from build123d import *

# Parameters (mm, degrees)
SKETCH1_R           = 4.7625
BOSS_EXTRUDE1_DEPTH = 12.7
SKETCH2_R           = 6.35
BOSS_EXTRUDE2_DEPTH = 50.8


with BuildPart() as part:
    # Sketch1 → Boss-Extrude1 (new body)
    with BuildSketch(Plane.XY):
        with BuildLine():
            Line((-12.7, 0), (-12.7, 127))
            Line((-12.7, 127), (12.7, 127))
            Line((12.7, 127), (12.7, 0))
            ThreePointArc((12.7, 0), (0, -12.7), (-12.7, 0))
        make_face()
        Circle(SKETCH1_R, mode=Mode.SUBTRACT)
    extrude(amount=BOSS_EXTRUDE1_DEPTH)

    # Sketch2 → Boss-Extrude2 (add)
    with BuildSketch(Plane(origin=(12.7, 0, 0), x_dir=(0, 0, -1), z_dir=(1, 0, 0))):
        with Locations((-6.35, 12.7)):
            Circle(SKETCH2_R)
    extrude(amount=BOSS_EXTRUDE2_DEPTH)


solid = part.part
Work out the finished part from the listing and answer in its coordinate system (mm). A direction names the side the tool comes from. Give positions to 0.01 mm unless a question says otherwise; leave off trailing zeros. Write each loop counter-clockwise with the first axis right and the second up, starting at its lowest first coordinate (ties: lowest second). Pieces come first, ordered by that corner, then holes. Notation, with made-up numbers: (27, 88.25) - (36, 88.25) arc R31 cw to (36, 119.25) - close; hole circle Ø11 at (14.25, 57.5). An arc over 180 degrees is marked (long way). One line per item, written item: value. Start each with the question number.
1. Consider probe 1 along Y at (x, z) = (0, 5.25); probe 2 along Y at (x, z) = (0.5, 4.75); probe 3 along X at (y, z) = (110.5, 3.5). Determine where each line is inside the solid, lowest interval first.
2. For a pull along X with two mould halves and no side action, classify faces 3 (the flat face through (12.7, 4, 6)), 4 (the flat face through (-12.7, 63, 6)), 5 (the cylindrical face through (-3.78, -2.9, 6.26)), 6 (the flat face through (0, 58, 12.7)) as +X half, -X half, draft (parallel to the pull), parting line (faces both ways), or undercut.
3. For faces 1 (the cylindrical face through (37.744, 18.054, 2.936)), 2 (the flat face through (63.5, 13, 6)), determine the directions among +Z, -Z, +X, -X, +Y, -Y from which every point of the face is accessible in a straight line to the end or side of a thin tool.
4. Find section D-D (y = 80). Write down the section's boundary in (x, z).
5. Find section C-C (y = -1.5). Write down the section's boundary in (x, z).
6. Find section A-A (x = 0). Write down the section's boundary in (y, z), then the cut area to 3 significant figures.
7. Given pin 1 (2 mm diameter, centred on y = 77, z = 11.5, fed in from +X); pin 2 (7.5 mm diameter, centred on x = 0, y = 0, fed in from -Z); pin 3 (6 mm diameter, centred on x = 49, z = 10, fed in from +Y), each flat-ended and moving along its own axis, determine where each tip first touches the part or whether it passes through.
Geometry results:
1. probe 1: -12.7 to -4.76, 4.76 to 127
1. probe 2: -12.69 to -4.74, 4.74 to 127
1. probe 3: -12.7 to 12.7
2. face 3: +X half
2. face 4: -X half
2. face 5: undercut
2. face 6: draft
3. face 1: +X
3. face 2: +Z, -Z, +X, +Y, -Y
4. outline: (-12.7, 0) - (12.7, 0) - (12.7, 12.7) - (-12.7, 12.7) - close
5. outline: (-12.61, 0) - (-4.52, 0) - (-4.52, 12.7) - (-12.61, 12.7) - close; (4.52, 0) - (12.61, 0) - (12.61, 12.7) - (4.52, 12.7) - close
6. outline: (-12.7, 0) - (-4.76, 0) - (-4.76, 12.7) - (-12.7, 12.7) - close; (4.76, 0) - (127, 0) - (127, 12.7) - (4.76, 12.7) - close
6. area: 1,650 mm2
7. pin 1: x = 12.7
7. pin 2: through
7. pin 3: y = 19.02
